The listing builds one solid part. Answer for the finished solid, in the listing's coordinates (mm). A direction names the side the tool comes from. Give positions to 0.01 mm unless a question says otherwise; leave off trailing zeros. Write each loop counter-clockwise with the first axis right and the second up, starting at its lowest first coordinate (ties: lowest second). Pieces come first, ordered by that corner, then holes.
Autodesk Inventor part; units mm, degrees
ref_plane "YZ Plane" through (0, 0, 0) normal (1, 0, 0) x (0, 1, 0)
ref_plane "XZ Plane" through (0, 0, 0) normal (0, 1, 0) x (-1, 0, 0)
ref_plane "XY Plane" through (0, 0, 0) normal (0, 0, 1) x (1, 0, 0)
sketch "Sketch1" plane through (0, 0, 0) normal (0, 1, 0) x (-1, 0, 0)
  line L0 (-10.16, 10.16) -> (10.16, 10.16)
  line L1 (10.16, 10.16) -> (10.16, -10.16)
  line L2 (-10.16, -10.16) -> (-10.16, 10.16)
  circle A0 centre (6.9088, -6.9148) radius 1.9304
  circle A1 centre (6.9088, 6.9088) radius 1.9304
  circle A2 centre (-6.9088, 6.9088) radius 1.9304
  circle A3 centre (-6.9088, -6.9148) radius 1.9304
  line L3 (-5.715, -10.16) -> (-5.715, -20.574)
  line L4 (-5.715, -20.574) -> (6.985, -20.574)
  line L5 (6.985, -20.574) -> (6.985, -10.16)
  line L6 (10.16, -10.16) -> (6.985, -10.16)
  line L7 (-5.715, -10.16) -> (-10.16, -10.16)
  point P0 (0, 0)
  dimension "d0" = 20.32
  dimension "d2" = 10.16
  dimension "d3" = 10.16
  dimension "d4" = 3.8608
  dimension "d5" = 6.9148
  dimension "d6" = 6.9088
  dimension "d7" = 3.8608
  dimension "d8" = 6.9088
  dimension "d9" = 6.9088
  dimension "d10" = 3.8608
  dimension "d11" = 6.9088
  dimension "d12" = 6.9088
  dimension "d13" = 3.8608
  dimension "d14" = 12.7
  dimension "d16" = 6.985
extrude "Extrusion1" add sketch "Sketch1" along normal blind 6.985
sketch "Sketch2" plane through (-6.985, 0, -20.574) normal (-1, 0, 0) x (0, 0, 1)
  circle A0 centre (5.08, 3.4925) radius 4.6609 construction
  line L0 (10.414, 0) -> (0, 0)
  line L1 (0, 0) -> (0, 6.985)
  line L2 (9.7409, 3.4925) -> (7.4105, -0.544)
  line L3 (7.4105, -0.544) -> (2.7496, -0.544)
  line L4 (2.7496, -0.544) -> (0.4191, 3.4925)
  line L5 (0.4191, 3.4925) -> (2.7495, 7.529)
  line L6 (2.7495, 7.529) -> (7.4104, 7.529)
  line L7 (7.4104, 7.529) -> (9.7409, 3.4925)
  point P0 (20.574, 0)
  dimension "d19" = 9.3218
  dimension "d20" = 3.4925
  dimension "d21" = 5.08
extrude "Extrusion2" cut sketch "Sketch2" against normal blind 3.81
sketch "Sketch3" plane through (5.715, 0, -10.16) normal (1, 0, 0) x (0, 0, -1)
  circle A0 centre (5.334, 3.4925) radius 1.9304
  line L0 (10.414, 0) -> (10.414, 6.985)
  line L1 (0, 6.985) -> (10.414, 6.985)
  point P0 (-10.16, 0)
  dimension "d24" = 3.8608
  dimension "d25" = 5.08
  dimension "d26" = 3.4925
extrude "Extrusion3" cut sketch "Sketch3" against normal through all
sketch "Sketch4" plane through (0, 6.985, 0) normal (0, 1, 0) x (1, 0, 0)
  circle A0 centre (0, 0) radius 6.35
  dimension "d29" = 12.7
extrude "Extrusion4" add sketch "Sketch4" along normal blind 2.54
sketch "Sketch5" plane through (0, 9.525, 0) normal (0, 1, 0) x (1, 0, 0)
  arc A0 (2.0472, -2.5908) -> (-2.0472, -2.5908) centre (0, 0) ccw
  line L0 (-2.0472, -2.5908) -> (2.0472, -2.5908)
  dimension "d32" = 6.604
  dimension "d33" = 2.5908
fillet "Fillet1" radius 3.3782 4 edges at (10.16, 3.4925, 10.16) (10.16, 3.4925, -10.16) (-10.16, 3.4925, 10.16) (-10.16, 3.4925, -10.16)
extrude "Extrusion5" cut sketch "Sketch5" against normal through all
sketch "Sketch6" plane through (0, 9.525, 0) normal (0, 1, 0) x (1, 0, 0)
  line L0 (-6.985, 20.574) -> (5.715, 20.574)
  line L1 (0.635, 0) -> (0.635, 20.574)
  line L2 (0.635, 20.574) -> (-0.635, 20.574)
  line L3 (-0.635, 20.574) -> (-0.635, 0)
  line L4 (-0.635, -20.574) -> (0.635, 20.574) construction
  line L5 (0.635, -20.574) -> (-0.635, 20.574) construction
  line L6 (-0.635, 0) -> (0.635, 0)
  point P0 (0, 0)
  dimension "d37" = 1.27
extrude "Extrusion6" cut sketch "Sketch6" against normal through all
sketch "Sketch7" plane through (0, 0, 0) normal (0, -1, 0) x (1, 0, 0)
  circle A0 centre (-6.9088, 6.9088) radius 1.9304 construction
  circle A1 centre (-6.9088, 6.9088) radius 4.6609 construction
  point P0 (0, 0)
  dimension "d40" = 9.3218
properties part number "clamping hub 1_4 D b"
Item 1: A cutting plane is placed at D-D, the plane z = -5.5. Give the vertices of the cut face in (x, y) (3 decimals).
Conclusion:
outline: (-10.16, 0) - (-8.222, 0) - (-8.222, 6.985) - (-10.16, 6.985) - close; (-5.595, 0) - (-0.635, 0) - (-0.635, 9.525) - (-3.174, 9.525) - (-3.174, 6.985) - (-5.595, 6.985) - close; (0.635, 0) - (5.595, 0) - (5.595, 6.985) - (3.174, 6.985) - (3.174, 9.525) - (0.635, 9.525) - close; (8.222, 0) - (10.16, 0) - (10.16, 6.985) - (8.222, 6.985) - close
Item 2: Consider probe 1 along Z at (x, y) = (-2.75, 3.75); probe 2 along X at (y, z) = (4.75, -11) (3 decimals); probe 3 along X at (y, z) = (6.25, -14.5) (3 decimals). Determine where each line is inside the solid, lowest interval first.
Conclusion:
probe 1: z = -20.57 to -17.41, -13.58 to -1.83, 1.83 to 10.16
probe 2: x = -6.985 to -0.635, 0.635 to 5.715
probe 3: x = -3.175 to -0.635, 0.635 to 5.715
Item 3: Each of these flat-tipped pins is pushed along its axis until it touches: P1, Ø3, axis at x = 7.5, z = -9, coming from the +Y side (3 decimals); P2, Ø5.5, axis at y = 2, z = -17.5, coming from the +X side (3 decimals); P3, Ø1, axis at x = 2, y = 8.5, coming from the +Z side. Where does it stop, or does it pass through?
Conclusion:
P1: stops at y = 6.985
P2: stops at x = 5.715
P3: stops at z = 6.17
Item 4: A cutting plane is placed at A-A, the plane z = 0. Give the vertices of the cut face in (x, y) (3 decimals), plus the area to 3 significant figures.
Conclusion:
outline: (-10.16, 0) - (-3.302, 0) - (-3.302, 9.525) - (-6.35, 9.525) - (-6.35, 6.985) - (-10.16, 6.985) - close; (3.302, 0) - (10.16, 0) - (10.16, 6.985) - (6.35, 6.985) - (6.35, 9.525) - (3.302, 9.525) - close
area: 111 mm2
Item 5: A cutting plane is placed at C-C, the plane x = -2.75. Give the vertices of the cut face in (y, z) (1 decimal), plus the area to 3 significant figures.
Conclusion:
outline: (0, -20.6) - (7, -20.6) - (7, -5.7) - (9.5, -5.7) - (9.5, -1.8) - (0, -1.8) - close; (0, 1.8) - (9.5, 1.8) - (9.5, 5.7) - (7, 5.7) - (7, 10.2) - (0, 10.2) - close; hole circle Ø3.9 at (3.5, -15.5)
area: 197 mm2
Item 6: Determine the mould class of faces 4 (the face through (-2, 0, -5)), 5 (the face through (-5.107, 5.214, -19.161)), 6 (the face through (9.14, 3.44, -9.2)) for opening direction Z: pulls with the +Z half, pulls with the -Z half, needs draft (parallel to the pull), parting line crosses it, or undercut.
Conclusion:
face 4: needs draft
face 5: undercut
face 6: pulls with the -Z half
Item 7: A cutting plane is placed at B-B, the plane y = 2. Count the separate pieces of the cut face and the enclosed holes in it, plus the area to 3 significant figures.
Conclusion:
separate pieces: 3
enclosed holes: 4
area: 387 mm2
Item 8: Which of the six approach directions +Z, -Z, +X, -X, +Y, -Y give full straight-line access (tool end or side, diameter ignored) to faces 1 (the face through (0, 5, 2.591)), 2 (the face through (0.635, 4, -12)), 3 (the face through (-4.4, 6.985, -5))?
Conclusion:
face 1: +Y, -Y
face 2: -Z, +Y, -Y
face 3: +Y
